Geometry check sheet. Reference: drawing and pictorial views, mm from the part's lowest x, y, z. Give positions to 0.01 mm unless a question says otherwise; leave off trailing zeros. Loops run counter-clockwise (first coordinate to the right, second up) from the corner with the lowest first, then second, coordinate; pieces in that order, holes last. Notation, with made-up numbers: (-29, -34) -> (10, -34) arc R7 ccw to (10, -30) -> close; hole circle Ø5 at (41.5, -17.75). An arc over 180 degrees is marked (long way). Answer in a Markdown table with one row per item. Add a question column.
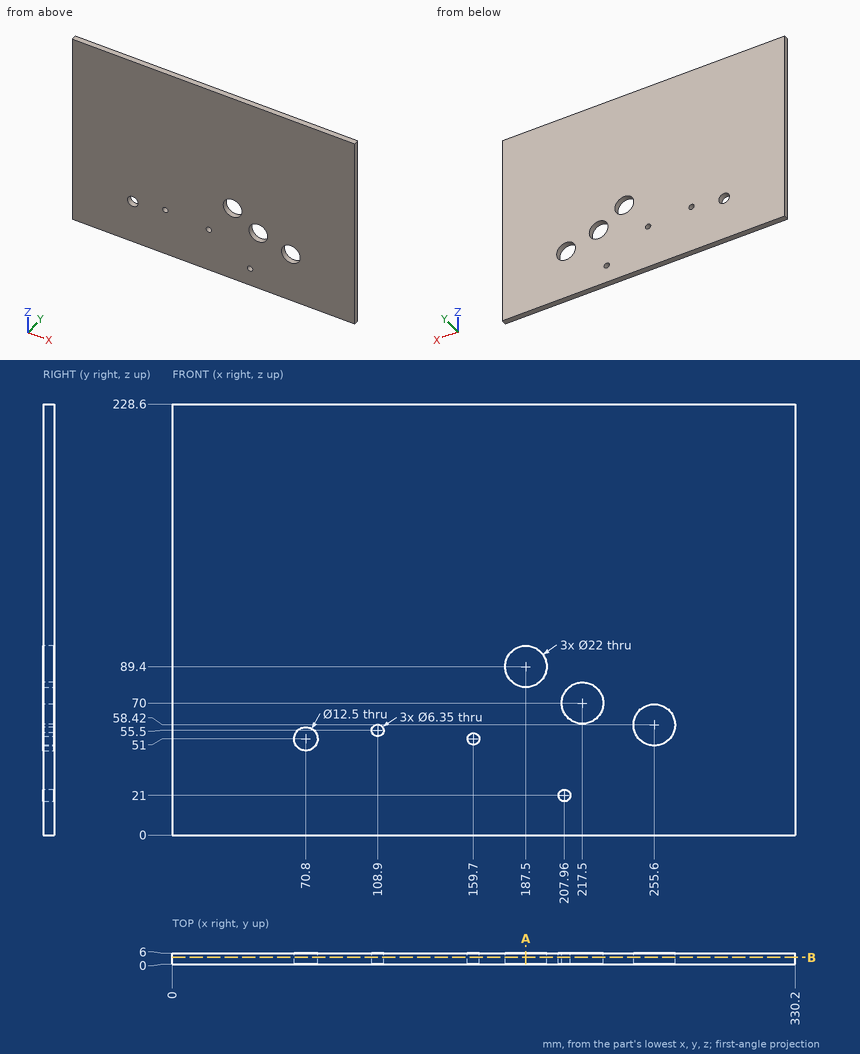
1. Sectioned sample at B-B (y = 3.7). Enter the section's corners in (x, z) (3 decimals), plus the area to 3 significant figures.
2. Sectioned sample at A-A (x = 187.5). Enter the section's corners in (y, z), plus the area to 3 significant figures.
3. Material ranges on L1, parallel to X at y = 4.65, z = 70; L2, parallel to X at y = 2.6, z = 58.42; L3, parallel to X at y = 3.15, z = 21 (3 decimals), recorded low to high. Write a range as from..to.
Response:
| question | item | result |
|---|---|---|
| 1 | outline | (0, 0) -> (330.2, 0) -> (330.2, 228.6) -> (0, 228.6) -> close; hole circle Ø12.5 at (70.8, 51); hole circle Ø6.35 at (108.9, 55.5); hole circle Ø6.35 at (159.7, 51); hole circle Ø22 at (187.5, 89.4); hole circle Ø6.35 at (207.96, 21); hole circle Ø22 at (217.5, 70); hole circle Ø22 at (255.6, 58.42) |
| 1 | area | 74,100 mm2 |
| 2 | outline | (0, 0) -> (6, 0) -> (6, 78.4) -> (0, 78.4) -> close; (0, 100.4) -> (6, 100.4) -> (6, 228.6) -> (0, 228.6) -> close |
| 2 | area | 1,240 mm2 |
| 3 | L1 | x = 0..206.5, 228.5..330.2 |
| 3 | L2 | x = 0..107.65, 110.15..244.6, 266.6..330.2 |
| 3 | L3 | x = 0..204.785, 211.135..330.2 |
